Can you work these out from the model? Positions are in its coordinate system, mm. Face numbers are marked on the shaded views. A direction names the side the tool comes from. Coordinates: 2 decimals unless noted, no trailing zeros. Loops run counter-clockwise (first coordinate to the right, second up) from the corner with the lowest first, then second, coordinate; pieces in that order, holes last. Notation, with made-up numbers: M 16,22 L 51,22 A22 cw 51,55 Z; hole C -13,82.5 d3. An arc over 180 degrees is marked long. Answer as a JSON object with one key per item and string values. Group by question number.
Item 1: If I drill on line 1 (Z direction, x = 1, y = -27); line 2 (Y direction, x = -14, z = 35); line 3 (Z direction, x = -18.5, y = -59), over which ranges is the centre line in solid material (lowest first)?
Item 2: Which directions (+Z, -Z, +X, -X, +Y, -Y) give clear straight access to the entire face, cutting with the end or side of a thin tool? Please do the marked faces 1 and 2.
Item 3: I'm going to push flat-ended pins straight in: pin 1 Ø8 at (x, z) = (-3, 138.5) entering from -Y; pin 2 Ø1.5 at (x, z) = (21, 109.5) entering from -Y; pin 3 Ø3 at (x, z) = (-1, 151.5) entering from -Y. Where does each tip first touch, or does it pass through?
Item 4: Suppose I cut it at C-C (z = 90). Write out the boundary of the cut face in (x, y).
Item 5: Suppose I cut it at D-D (y = -64.5). Write out the boundary of the cut face in (x, z), then the cut area to 3 significant figures.
Item 6: Suppose I cut it at B-B (x = 0). Write out the boundary of the cut face in (y, z).
Item 7: Suppose I cut it at A-A (y = -36). Write out the boundary of the cut face in (x, z), then the cut area to 3 significant figures.
Item 8: We'd pull the mould along Z, two halves only. Please class the marked faces 3, 4 and 5: +Z half, -Z half, draft (parallel to the pull), parting line (faces both ways), or undercut.
```python
from build123d import *

# Parameters (mm, degrees)
F0_W     = 76.2
F0_H     = 8.382
F1_DEPTH = 76.2
F2_W     = 38.1
F2_H     = 152.4
F3_DEPTH = 7.62
F4_W     = 38.1
F4_H     = 38.1
F5_DEPTH = 6.35


with BuildPart() as f1:
    # F0 (on Front) → F1 (new body)
    with BuildSketch(Plane.XZ):
        Rectangle(F0_W, F0_H)
    extrude(amount=F1_DEPTH)

    # F2 (on Front) → F3 (join)
    with BuildSketch(Plane.XZ):
        with Locations((0, 72.009)):
            Rectangle(F2_W, F2_H)
    extrude(amount=F3_DEPTH)

    # F4 (on face) → F5 (join)
    with BuildSketch(Plane.XY.offset(148.209)):
        with Locations((0, -19.05)):
            Rectangle(F4_W, F4_H)
    extrude(amount=F5_DEPTH)


solid = f1.part
```
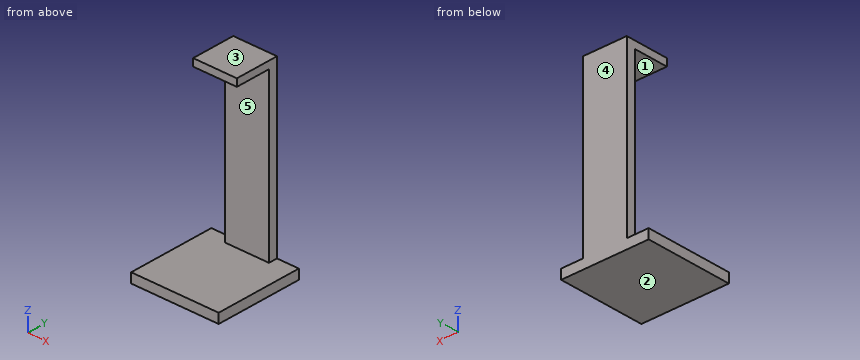
From the geometry:
{
 "1": {"line 1": "-4.19 to 4.19, 148.21 to 154.56", "line 2": "-7.62 to 0", "line 3": "-4.19 to 4.19"},
 "2": {"face 1": "+X, -X, -Y", "face 2": "-Z, +X, -X, +Y, -Y"},
 "3": {"pin 1": "y = -7.62", "pin 2": "through", "pin 3": "y = -38.1"},
 "4": {"outline": "M -19.05,-7.62 L 19.05,-7.62 L 19.05,0 L -19.05,0 Z"},
 "5": {"outline": "M -38.1,-4.19 L 38.1,-4.19 L 38.1,4.19 L -38.1,4.19 Z", "area": "639 mm2"},
 "6": {"outline": "M -76.2,-4.19 L 0,-4.19 L 0,154.56 L -38.1,154.56 L -38.1,148.21 L -7.62,148.21 L -7.62,4.19 L -76.2,4.19 Z"},
 "7": {"outline": "M -38.1,-4.19 L 38.1,-4.19 L 38.1,4.19 L -38.1,4.19 Z; M -19.05,148.21 L 19.05,148.21 L 19.05,154.56 L -19.05,154.56 Z", "area": "881 mm2"},
 "8": {"face 3": "+Z half", "face 4": "draft", "face 5": "undercut"}
}
